Part model, mm, in its own coordinate system. A direction names the side the tool comes from. Coordinates: 2 decimals unless noted, no trailing zeros. Order: outer loops, then holes, each group sorted by start corner. A loop starts at its lowest first (then second) coordinate and runs counter-clockwise, first axis right, second up.
from build123d import *

# Parameters (mm, degrees)
SKETCH_1_W          = 42
SKETCH_1_H          = 42
EXTRUDE_1_DEPTH     = 21
CHAMFER_1_SIZE      = 4
SKETCH_2_R          = 18
EXTRUDE_2_DEPTH     = 30
SKETCH_3_R          = 4
EXTRUDE_3_DEPTH     = 20
CUT_EXTRUDE_START   = -15
CUT_EXTRUDE_1_DEPTH = 15


with BuildPart() as part:
    # 스케치1 → 보스-돌출1 (new, symmetric)
    with BuildSketch(Plane(origin=(0, 0, 0), x_dir=(1, 0, 0), z_dir=(0, 1, 0))):
        Rectangle(SKETCH_1_W, SKETCH_1_H)
    extrude(amount=EXTRUDE_1_DEPTH, both=True)

    # 모따기1
    chamfer_1_edges = [part.edges().sort_by_distance(p)[0] for p in [
        (21, 0, 21),
        (-21, 0, 21),
        (-21, 0, -21),
        (21, 0, -21),
    ]]
    chamfer(chamfer_1_edges, length=CHAMFER_1_SIZE)

    # 스케치2 → 보스-돌출2 (add)
    with BuildSketch(Plane(origin=(0, 21, 0), x_dir=(1, 0, 0), z_dir=(0, 1, 0))):
        with Locations(Location((0, 0, 0), (0, 0, 270))):
            Circle(SKETCH_2_R)
    extrude(amount=EXTRUDE_2_DEPTH)

    # 스케치3 → 보스-돌출3 (add)
    with BuildSketch(Plane(origin=(0, 51, 0), x_dir=(1, 0, 0), z_dir=(0, 1, 0))):
        with Locations(Location((0, 0, 0), (0, 0, 270))):
            Circle(SKETCH_3_R)
    extrude(amount=EXTRUDE_3_DEPTH)

    # 스케치4 → 컷-돌출1 (cut)
    with BuildSketch(Plane(origin=(0, 71, 0), x_dir=(1, 0, 0), z_dir=(0, 1, 0)).offset(CUT_EXTRUDE_START)):
        with BuildLine():
            Line((-2.645751311, 3), (2.645751311, 3))
            ThreePointArc((2.645751311, 3), (0, 4), (-2.645751311, 3))
        make_face()
    extrude(amount=CUT_EXTRUDE_1_DEPTH, mode=Mode.SUBTRACT)


solid = part.part
Q1. Cut at A-A on y = 5. Write the cut outline in (x, z), and give its area (3 significant figures).
Results list:
outline: (-21, -17) - (-17, -21) - (17, -21) - (21, -17) - (21, 17) - (17, 21) - (-17, 21) - (-21, 17) - close
area: 1,730 mm2
Q2. Cut at D-D on z = 12. Write the cut outline in (x, y).
Results list:
outline: (-21, -21) - (21, -21) - (21, 21) - (13.42, 21) - (13.42, 51) - (-13.42, 51) - (-13.42, 21) - (-21, 21) - close
Q3. Cut at C-C on z = 0. Write the cut outline in (x, y), and give its area (3 significant figures).
Results list:
outline: (-21, -21) - (21, -21) - (21, 21) - (18, 21) - (18, 51) - (4, 51) - (4, 71) - (-4, 71) - (-4, 51) - (-18, 51) - (-18, 21) - (-21, 21) - close
area: 3,000 mm2
Q4. Pin check, flat tips, straight feed: pin 1 Ø1 at (x, z) = (11.5, -16) entering from +Y; pin 2 Ø1.6 at (x, y) = (-1, 66) entering from -Z; pin 3 Ø1 at (x, y) = (-0.5, 25) entering from -Z. Stop position of each tip, or through.
Results list:
pin 1: stops at y = 21
pin 2: stops at z = -3
pin 3: stops at z = -18
Q5. Wall check: line 1 along Y through (x, z) = (-2, -4.5); line 2 along Y through (x, z) = (16.5, -9.5); line 3 along Z through (x, y) = (0.5, 53.5). Give the ranges that are in metal, low to high.
Results list:
line 1: y = -21 to 51
line 2: y = -21 to 21
line 3: z = -3.97 to 3.97
Q6. Cut at B-B on x = 0. Write the cut outline in (y, z).
Results list:
outline: (-21, -21) - (21, -21) - (21, -18) - (51, -18) - (51, -4) - (56, -4) - (56, -3) - (71, -3) - (71, 4) - (51, 4) - (51, 18) - (21, 18) - (21, 21) - (-21, 21) - close
Q7. Which spindle directions (+Z, -Z, +X, -X, +Y, -Y) get a long thin tool onto all of the face, cutting with end or side? Do faces 1 (the face through (-19, 0, -19)), 2 (the face through (1.201, 60.86, 3.815)), 3 (the face through (0, 63, -3)). Say none if no direction does.
Results list:
face 1: -Z, -X, +Y, -Y
face 2: +Y
face 3: -Z, +X, -X, +Y
